CAD build for the part. Positions are in the model's coordinates, mm. Face numbers are marked on the shaded views. A direction names the side the tool comes from. Coordinates: 2 decimals unless noted, no trailing zeros. Order: outer loops, then holes, each group sorted by start corner. A loop starts at its lowest first (then second) coordinate and runs counter-clockwise, first axis right, second up. Notation, with made-up numbers: (58.5, 88) -> (70.5, 88) arc R27 ccw to (70.5, 122) -> close; hole circle Ø10 at (86.5, 83.25). An arc over 180 degrees is marked (long way). Use one line per item in the form item = value. Start each with the question number.
from build123d import *

# Parameters (mm, degrees)
BOSS_EXTRUDE1_DEPTH = 8
CUT_EXTRUDE1_DEPTH  = 8
SKETCH4_R           = 2.5
BOSS_EXTRUDE2_DEPTH = 5


with BuildPart() as part:
    # Sketch1 → Boss-Extrude1 (new body)
    with BuildSketch(Plane(origin=(0, 0, 0), x_dir=(0, 1, 0), z_dir=(0, 0, 1))):
        with BuildLine():
            Line((-12, 3.5), (-5.595533933, 3.5))
            ThreePointArc((-5.595533933, 3.5), (6.6, 0), (-5.595533933, -3.5))
            Line((-5.595533933, -3.5), (-12, -3.5))
            Line((-12, -3.5), (-12, -0.5))
            Line((-12, -0.5), (-4.06939799, -0.5))
            ThreePointArc((-4.06939799, -0.5), (4.1, 0), (-4.06939799, 0.5))
            Line((-4.06939799, 0.5), (-12, 0.5))
            Line((-12, 0.5), (-12, 3.5))
        make_face()
    extrude(amount=BOSS_EXTRUDE1_DEPTH)

    # Sketch2 → Cut-Extrude1 (cut)
    with BuildSketch(Plane(origin=(-3.5, 0, 0), x_dir=(0, -1, 0), z_dir=(-1, 0, 0))):
        with BuildLine():
            ThreePointArc((10.297766967, 4), (9.858427138, 5.060660172), (8.797766967, 5.5))
            Line((8.797766967, 5.5), (8.797766967, 2.5))
            ThreePointArc((8.797766967, 2.5), (9.858427138, 2.939339828), (10.297766967, 4))
        make_face()
        with BuildLine():
            Line((8.797766967, 2.5), (8.797766967, 5.5))
            ThreePointArc((8.797766967, 5.5), (7.297766967, 4), (8.797766967, 2.5))
        make_face()
    extrude(amount=-CUT_EXTRUDE1_DEPTH, mode=Mode.SUBTRACT)

    # Sketch4 → Boss-Extrude2 (add)
    # profile 1 of 2: a face of its own
    with BuildSketch(Plane(origin=(0, 0, 0), x_dir=(1, 0, 0), z_dir=(0, 0, -1))):
        with BuildLine():
            Line((20, 5.595533933), (14, 5.595533933))
            Line((14, 5.595533933), (4.863001587, 4.462198513))
            ThreePointArc((4.863001587, 4.462198513), (6.540217456, -0.886315759), (3.5, -5.595533933))
            Line((3.5, -5.595533933), (20, -5.595533933))
            Line((20, -5.595533933), (20, 5.595533933))
        make_face()
        with Locations(Location((14, 0, 0), (0, 0, 180))):
            Circle(SKETCH4_R, mode=Mode.SUBTRACT)
    # profile 2 of 2: a face of its own
    with BuildSketch(Plane(origin=(0, 0, 0), x_dir=(1, 0, 0), z_dir=(0, 0, -1))):
        with BuildLine():
            Line((-20, -5.595533933), (-3.5, -5.595533933))
            ThreePointArc((-3.5, -5.595533933), (-6.540217456, -0.886315759), (-4.863001587, 4.462198513))
            Line((-4.863001587, 4.462198513), (-14, 5.595533933))
            Line((-14, 5.595533933), (-20, 5.595533933))
            Line((-20, 5.595533933), (-20, -5.595533933))
        make_face()
        with Locations(Location((-13.139356118, 0, 0), (0, 0, 180))):
            Circle(SKETCH4_R, mode=Mode.SUBTRACT)
    extrude(amount=-BOSS_EXTRUDE2_DEPTH)


solid = part.part
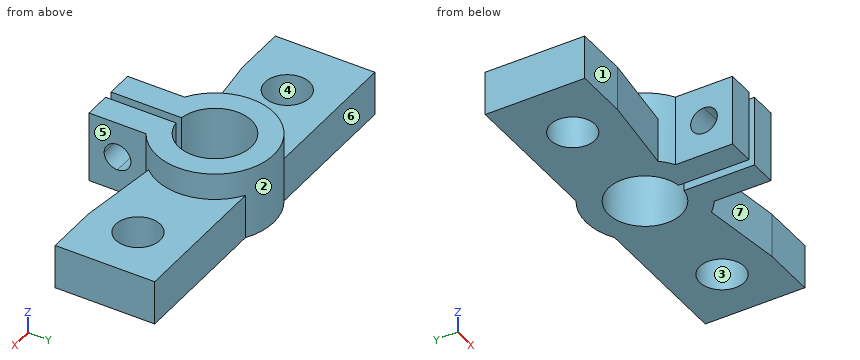
1) Drop flat-ended pins along their axis: P1, Ø3, axis at x = 14, y = 0, coming from the +Z side; P2, Ø4, axis at x = -16, z = 1.5, coming from the +Y side; P3, Ø1.9, axis at y = -9.5, z = 5.5, coming from the -X side; P4, Ø3.5, axis at x = -9.5, y = -1.5, coming from the +Z side. Give the stop position or say it passes through.
2) Two-plate mould, pull along Y, no slides. Class the marked faces 1, 2, 3 and 4: released by +Y, released by -Y, zero draft, split by the parting line, or undercut.
3) Probe L1, parallel to Y at x = 14, z = 1.9; L2, parallel to X at y = -10.75, z = 2; L3, parallel to X at y = 0.5, z = 2.5. List the from-to ranges inside material, lowest first.
4) Cut at A-A on y = 0. Give the cut face in (x, z), then the cut area to 3 significant figures.
5) 3-axis set-ups, long thin cutter, end or side, ignore diameter. For the marked faces 5, 6 and 7: which of +Z, -Z, +X, -X, +Y, -Y reach the whole face in a straight line?
6) Cut at B-B on z = 3.5. Give the cut face in (x, y).
7) Cut at C-C on z = 6.25. Give the cut face in (x, y).
8) Cut at D-D on z = 1. Give the cut face in (x, y), then the cut area to 3 significant figures.
Values follow:
q1.P1 = through
q1.P2 = 5.6
q1.P3 = -3.5
q1.P4 = 5
q2.face_1 = released by -Y
q2.face_2 = split by the parting line
q2.face_3 = undercut
q2.face_4 = undercut
q3.L1 = -5.6 to -2.5, 2.5 to 5.6
q3.L2 = -3.5 to -0.5, 0.5 to 3.5
q3.L3 = -20 to -15.59, -10.69 to -4.07, 4.07 to 11.55, 16.45 to 20
q4.outline = (-20, 0) -> (-15.64, 0) -> (-15.64, 5) -> (-20, 5) -> close; (-10.64, 0) -> (-4.1, 0) -> (-4.1, 8) -> (-6.6, 8) -> (-6.6, 5) -> (-10.64, 5) -> close; (4.1, 0) -> (11.5, 0) -> (11.5, 5) -> (6.6, 5) -> (6.6, 8) -> (4.1, 8) -> close; (16.5, 0) -> (20, 0) -> (20, 5) -> (16.5, 5) -> close
q4.area = 124 mm^2
q5.face_5 = +Z, -Z, +X, -Y
q5.face_6 = +Z, -Z, -X, +Y
q5.face_7 = +Z, -Z, -Y
q6.outline = (-20, -5.6) -> (-14, -5.6) -> (-4.86, -4.46) arc R6.6 ccw to (-3.5, -5.6) -> (-3.5, -7.38) -> (-0.5, -7.38) -> (-0.5, -4.07) arc R4.1 cw (long way) to (0.5, -4.07) -> (0.5, -7.38) -> (3.5, -7.38) -> (3.5, -5.6) arc R6.6 ccw to (4.86, -4.46) -> (14, -5.6) -> (20, -5.6) -> (20, 5.6) -> (3.5, 5.6) arc R6.6 ccw to (-3.5, 5.6) -> (-20, 5.6) -> close; (-3.5, -12) -> (-0.5, -12) -> (-0.5, -10.21) -> (-3.5, -10.21) -> close; (0.5, -12) -> (3.5, -12) -> (3.5, -10.21) -> (0.5, -10.21) -> close; hole circle Ø5 at (-13.14, 0); hole circle Ø5 at (14, 0)
q7.outline = (-3.5, -12) -> (-0.5, -12) -> (-0.5, -4.07) arc R4.1 cw (long way) to (0.5, -4.07) -> (0.5, -12) -> (3.5, -12) -> (3.5, -5.6) arc R6.6 ccw (long way) to (-3.5, -5.6) -> close
q8.outline = (-20, -5.6) -> (-14, -5.6) -> (-4.86, -4.46) arc R6.6 ccw to (-3.5, -5.6) -> (-3.5, -12) -> (-0.5, -12) -> (-0.5, -4.07) arc R4.1 cw (long way) to (0.5, -4.07) -> (0.5, -12) -> (3.5, -12) -> (3.5, -5.6) arc R6.6 ccw to (4.86, -4.46) -> (14, -5.6) -> (20, -5.6) -> (20, 5.6) -> (3.5, 5.6) arc R6.6 ccw to (-3.5, 5.6) -> (-20, 5.6) -> close; hole circle Ø5 at (-13.14, 0); hole circle Ø5 at (14, 0)
q8.area = 385 mm^2
